```python
from build123d import *

# Parameters (mm, degrees)
F0_W     = 56.9933205843
F0_H     = 84.123885259
F1_DEPTH = 71.59423
F2_R     = 14.1167569705
F3_DEPTH = 25.4
F4_W     = 28.7987589836
F4_H     = 43.1953351945
F5_DEPTH = 25.4


with BuildPart() as f1:
    # F0 (on Front) → F1 (new body)
    with BuildSketch(Plane.XZ):
        with Locations((-84.2327773571, 12.7716520801)):
            Rectangle(F0_W, F0_H)
    extrude(amount=F1_DEPTH)

    # F2 (on face) → F3 (cut)
    with BuildSketch(Plane.YZ.offset(-55.736117065)):
        with Locations((-35.797115, 12.7716520801)):
            Circle(F2_R)
    extrude(amount=-F3_DEPTH, mode=Mode.SUBTRACT)

    # F4 (on face) → F5 (join)
    with BuildSketch(Plane.XZ.offset(71.59423)):
        with Locations((-84.2327773571, 12.7716520801)):
            Rectangle(F4_W, F4_H)
    extrude(amount=F5_DEPTH)


solid = f1.part
```
CAD build for the part. Positions are in the model's coordinates, mm. A direction names the side the tool comes from. Coordinates: 2 decimals unless noted, no trailing zeros. Write each loop counter-clockwise with the first axis right and the second up, starting at its lowest first coordinate (ties: lowest second). Pieces come first, ordered by that corner, then holes.
(1) Cut at C-C, the plane x = -80. List the corners of the cut face in (y, z), and give its area (3 significant figures).
(2) Cut at B-B, the plane z = 16.5. List the corners of the cut face in (x, y), and give its area (3 significant figures).
(3) 3-axis set-ups, long thin cutter, end or side, ignore diameter. For faces 1 (the face through (-98.632, -84, 12)), 2 (the face through (-68.3, -49.9, 13.4)), 3 (the face through (-69.833, -84, 12)), 4 (the face through (-84, -84, 34.369)), 5 (the face through (-85, -35, 54.834)): which of +Z, -Z, +X, -X, +Y, -Y reach the whole face in a straight line?
(4) Drill centre lines: probe 1 along Y at (x, z) = (-71.5, -22.5); probe 2 along Z at (x, y) = (-92.5, -82); probe 3 along X at (y, z) = (-78, 6.5). Where is each one in solid material? Low to high.
(5) Flat gauge pins, fed straight in: pin 1 (20.5 mm diameter, centred on y = -87, z = 22.5, fed in from -X); pin 2 (7.5 mm diameter, centred on x = -84, y = -89.5, fed in from +Z); pin 3 (2 mm diameter, centred on x = -73.5, z = 40, fed in from -Y). Where does each tip first touch, or does it go through?
(6) Cut at D-D, the plane y = -78. List the corners of the cut face in (x, z), and give its area (3 significant figures).
(7) Two-plate mould, pull along Z, no slides. Class faces 6 (the face through (-84, -84, -8.826)), 7 (the face through (-104, -71.594, 13)), 8 (the face through (-81.136, -36, 13)): +Z half, -Z half, draft (parallel to the pull), parting line (faces both ways), or undercut.
(8) Cut at A-A, the plane x = -90.5. List the corners of the cut face in (y, z).
Geometry says:
1. outline: (-96.99, -8.83) - (-71.59, -8.83) - (-71.59, -29.29) - (0, -29.29) - (0, 54.83) - (-71.59, 54.83) - (-71.59, 34.37) - (-96.99, 34.37) - close; hole circle Ø28.23 at (-35.8, 12.77)
1. area: 6,490 mm2
2. outline: (-112.73, -71.59) - (-98.63, -71.59) - (-98.63, -96.99) - (-69.83, -96.99) - (-69.83, -71.59) - (-55.74, -71.59) - (-55.74, -49.41) - (-81.14, -49.41) - (-81.14, -22.18) - (-55.74, -22.18) - (-55.74, 0) - (-112.73, 0) - close
2. area: 4,120 mm2
3. face 1: +Z, -Z, -X, -Y
3. face 2: +X
3. face 3: +Z, -Z, +X, -Y
3. face 4: +Z, +X, -X, -Y
3. face 5: +Z, +X, -X, +Y, -Y
4. probe 1: y = -71.59 to 0
4. probe 2: z = -8.83 to 34.37
4. probe 3: x = -98.63 to -69.83
5. pin 1: stops at x = -98.63
5. pin 2: stops at z = 34.37
5. pin 3: stops at y = -71.59
6. outline: (-98.63, -8.83) - (-69.83, -8.83) - (-69.83, 34.37) - (-98.63, 34.37) - close
6. area: 1,240 mm2
7. face 6: -Z half
7. face 7: draft
7. face 8: undercut
8. outline: (-96.99, -8.83) - (-71.59, -8.83) - (-71.59, -29.29) - (0, -29.29) - (0, 54.83) - (-71.59, 54.83) - (-71.59, 34.37) - (-96.99, 34.37) - close
